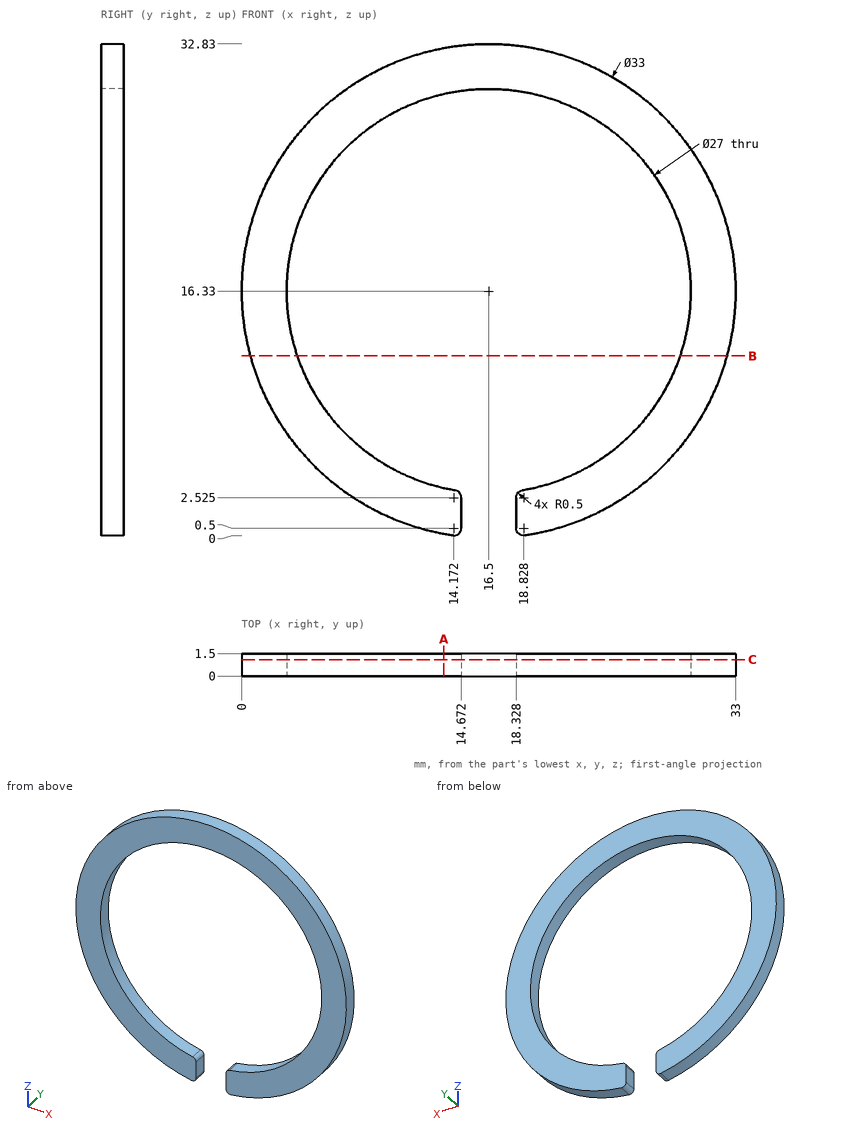
The drawing under review shows one solid part. Ordinate dimensions are in mm from its lowest x, y, z. Give positions to 0.01 mm unless a question says otherwise; leave off trailing zeros. Write each loop counter-clockwise with the first axis right and the second up, starting at its lowest first coordinate (ties: lowest second). Pieces come first, ordered by that corner, then holes.
1. Add section C-C, the plane y = 1.1. Write out the cut boundary in (x, z) (1 decimal).
2. Add section B-B, the plane z = 12. Write out the cut boundary in (x, y).
3. Add section A-A, the plane x = 13.5. Write out the cut boundary in (y, z) (1 decimal).
4. Wall thickness on L1, parallel to X at y = 0.9, z = 16.5; L2, parallel to X at y = 0.75, z = 12; L3, parallel to Z at x = 26.5, y = 0.7 (1 decimal): over which ranges is each line inside the solid? List them lowest first.
Worked answers:
1. outline: (14.1, 0) arc R0.5 ccw to (14.7, 0.5) - (14.7, 2.5) arc R0.5 ccw to (14.3, 3) arc R13.5 cw (long way) to (18.7, 3) arc R0.5 ccw to (18.3, 2.5) - (18.3, 0.5) arc R0.5 ccw to (18.9, 0) arc R16.5 ccw (long way) to start
2. outline: (0.58, 0) - (3.71, 0) - (3.71, 1.5) - (0.58, 1.5) - close; (29.29, 0) - (32.42, 0) - (32.42, 1.5) - (29.29, 1.5) - close
3. outline: (0, 0.1) - (1.5, 0.1) - (1.5, 3.2) - (0, 3.2) - close; (0, 29.5) - (1.5, 29.5) - (1.5, 32.6) - (0, 32.6) - close
4. L1: x = 0 to 3, 30 to 33
4. L2: x = 0.58 to 3.71, 29.29 to 32.42
4. L3: z = 3.2 to 7.3, 25.4 to 29.5
